Can you work these out from the model? Positions are in its coordinate system, mm. A direction names the side the tool comes from. Coordinates: 2 decimals unless noted, no trailing zeros. Loops run counter-clockwise (first coordinate to the right, second up) from the corner with the lowest first, then second, coordinate; pieces in that order, holes last.
```python
from build123d import *

# Parameters (mm, degrees)
SKETCH1_W           = 104
SKETCH1_H           = 62
BOSS_EXTRUDE1_DEPTH = 5
CUT_EXTRUDE1_DEPTH  = 10


with BuildPart() as part:
    # Sketch1 → Boss-Extrude1 (new body)
    with BuildSketch(Plane.XY):
        Rectangle(SKETCH1_W, SKETCH1_H)
    extrude(amount=BOSS_EXTRUDE1_DEPTH)

    # Sketch2 → Cut-Extrude1 (cut)
    with BuildSketch(Plane(origin=(0, 0, 0), x_dir=(-1, 0, 0), z_dir=(0, 0, -1))):
        Polygon((-37.6, -28), (-37.6, -31), (-42, -31), (-42, -28), (-43.5, -28), (-43.5, -24.6), (-42, -24.6), (-42, -10.8), (-37.6, -10.8), (-37.6, -24.6), (-36.1, -24.6), (-36.1, -28), align=None)
        Polygon((42, -31), (42, -28), (43.5, -28), (43.5, -24.6), (42, -24.6), (42, -10.8), (37.6, -10.8), (37.6, -24.6), (36.1, -24.6), (36.1, -28), (37.6, -28), (37.6, -31), align=None)
        Polygon((-42, 31), (-42, 28), (-43.5, 28), (-43.5, 24.6), (-42, 24.6), (-42, 10.8), (-37.6, 10.8), (-37.6, 24.6), (-36.1, 24.6), (-36.1, 28), (-37.6, 28), (-37.6, 31), align=None)
        Polygon((14.4, 13.8), (14.4, 10.8), (10, 10.8), (10, 13.8), (8.5, 13.8), (8.5, 17.2), (10, 17.2), (10, 31), (14.4, 31), (14.4, 17.2), (15.9, 17.2), (15.9, 13.8), align=None)
    extrude(amount=-CUT_EXTRUDE1_DEPTH, mode=Mode.SUBTRACT)


solid = part.part
```
(1) I want a section at A-A on y = -12. Write out the boundary of the cut face in (x, z).
Check values:
outline: (-52, 0) - (-42, 0) - (-42, 5) - (-52, 5) - close; (-37.6, 0) - (37.6, 0) - (37.6, 5) - (-37.6, 5) - close; (42, 0) - (52, 0) - (52, 5) - (42, 5) - close
(2) If I drill on probe 1 along X at (y, z) = (-16, 1.05); probe 2 along X at (y, z) = (11, 1.35); probe 3 along Y at (x, z) = (-43, 2.15), over which ranges is the centre line in solid material (lowest first)?
Check values:
probe 1: x = -52 to -42, -37.6 to 37.6, 42 to 52
probe 2: x = -52 to -14.4, -10 to 37.6, 42 to 52
probe 3: y = -31 to -28, -24.6 to 31
(3) If we mould it in two halves opening along Y, with no side actions, what happens to faces 1 (the flat face through (-42, -30, 2)), 2 (the flat face through (47, -31, 2)), 3 (the flat face through (-43.5, -26, 2))? For each: released by +Y, released by -Y, zero draft, split by the parting line, or undercut.
Check values:
face 1: zero draft
face 2: released by -Y
face 3: undercut
(4) I want a section at B-B on y = 15.5. Write out the boundary of the cut face in (x, z), then the cut area to 3 significant figures.
Check values:
outline: (-52, 0) - (-15.9, 0) - (-15.9, 5) - (-52, 5) - close; (-8.5, 0) - (37.6, 0) - (37.6, 5) - (-8.5, 5) - close; (42, 0) - (52, 0) - (52, 5) - (42, 5) - close
area: 461 mm2
(5) Which directions (+Z, -Z, +X, -X, +Y, -Y) give clear straight access to the entire face, cutting with the end or side of a thin tool? Please do faces 4 (the flat face through (-36.1, -26, 2)), 5 (the flat face through (-1, 0, 0)), 6 (the flat face through (37.6, -29, 2)), 7 (the flat face through (37.6, 18, 2)).
Check values:
face 4: +Z, -Z
face 5: -Z, +X, -X, +Y, -Y
face 6: +Z, -Z, -Y
face 7: +Z, -Z, +Y
